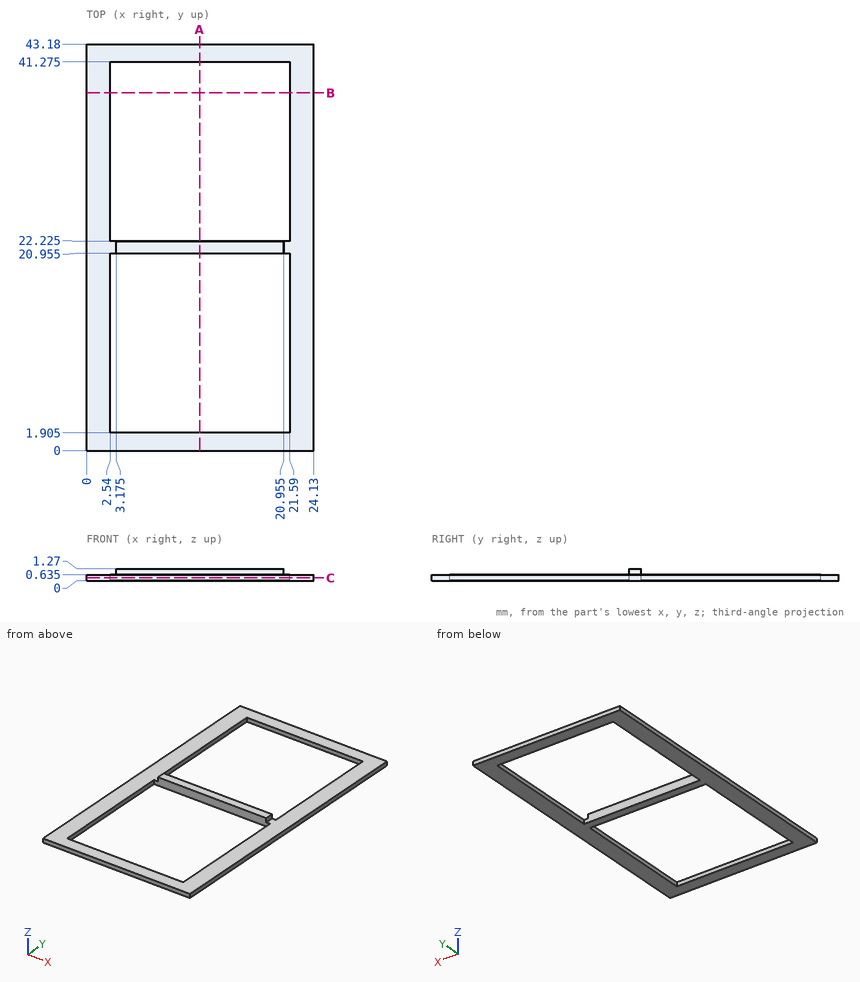
Geometry check sheet. Reference: drawing and pictorial views, mm from the part's lowest x, y, z. Round coordinates to 2 decimals unless told otherwise and drop trailing zeros. Order: outer loops, then holes, each group sorted by start corner. A loop starts at its lowest first (then second) coordinate and runs counter-clockwise, first axis right, second up. Notation, with made-up numbers: (82.25, 85) -> (107.25, 85) arc R14 ccw to (107.25, 89) -> close; hole circle Ø4 at (10, 50.5). An arc over 180 degrees is marked (long way). One line per item, written item: value. Start each with the question number.
Q1. Cross-section at B-B (y = 38). Record the boundary of the cut face in (x, z) (3 decimals).
Q2. Thickness scan on line 1 (Y direction, x = 19.75, z = 0.4) (3 decimals); line 2 (X direction, y = 23, z = 0.2); line 3 (Y direction, x = 3.75, z = 0.85) (3 decimals). Record the ranges inside material, lowest first.
Q3. Gauge pin test, flat end, axial feed: pin 1 Ø10 at (x, y) = (16.5, 35) entering from -Z. Record the tip position at first contact, or that the pin passes through.
Q4. Cross-section at C-C (z = 0.3). Record the boundary of the cut face in (x, y) (3 decimals).
Q5. Cross-section at A-A (x = 12). Record the boundary of the cut face in (y, z) (3 decimals).
Completed:
1. outline: (0, 0) -> (2.54, 0) -> (2.54, 0.635) -> (0, 0.635) -> close; (21.59, 0) -> (24.13, 0) -> (24.13, 0.635) -> (21.59, 0.635) -> close
2. line 1: y = 0 to 1.905, 20.955 to 22.225, 41.275 to 43.18
2. line 2: x = 0 to 2.54, 21.59 to 24.13
2. line 3: y = 20.955 to 22.225
3. pin 1: passes through
4. outline: (0, 0) -> (24.13, 0) -> (24.13, 43.18) -> (0, 43.18) -> close; hole (2.54, 1.905) -> (21.59, 1.905) -> (21.59, 20.955) -> (2.54, 20.955) -> close; hole (2.54, 22.225) -> (21.59, 22.225) -> (21.59, 41.275) -> (2.54, 41.275) -> close
5. outline: (0, 0) -> (1.905, 0) -> (1.905, 0.635) -> (0, 0.635) -> close; (20.955, 0) -> (22.225, 0) -> (22.225, 1.27) -> (20.955, 1.27) -> close; (41.275, 0) -> (43.18, 0) -> (43.18, 0.635) -> (41.275, 0.635) -> close
